Check sheet for the modelled part. Datum: model origin and axes. Units: mm. Face numbers are marked on the shaded views. A direction names the side the tool comes from. Coordinates: 2 decimals unless noted, no trailing zeros. Write each loop counter-clockwise with the first axis right and the second up, starting at its lowest first coordinate (ties: lowest second). Pieces come first, ordered by that corner, then holes. Notation, with made-up numbers: (51, 85.25) - (81, 85.25) arc R33 ccw to (81, 124.25) - close; hole circle Ø8 at (85.25, -13.5). An arc over 180 degrees is marked (long way). Use one line per item in the form item = value. Start each with the question number.
1. Cross-section at A-A on z = 4.5. Record the boundary of the cut face in (x, y).
2. Go/stop test with flat-tipped pins: pin 1 Ø2 at (y, z) = (53.5, 6.5) entering from -X; pin 2 Ø6 at (x, z) = (-11, 10) entering from +Y; pin 3 Ø10 at (x, z) = (-10, 8) entering from -Y. Record where each tip stops, or that it passes through.
3. Cross-section at C-C on y = 6.5. Record the boundary of the cut face in (x, z), then the cut area to 3 significant figures.
4. Tool access check on the marked faces 1, 2 and 3. Record the directions out of +Z, -Z, +X, -X, +Y, -Y that give a thin tool (end or side, any length) a straight path to the whole face; none if there is none.
5. Scan lines: line 1 along X through (y, z) = (51.5, 8); line 2 along Y through (x, z) = (25, 3.75). Record each from-to range of solid material in increasing order.
6. Cross-section at B-B on x = 25. Record the boundary of the cut face in (y, z), then the cut area to 3 significant figures.
```python
from build123d import *

# Parameters (mm, degrees)
F0_W     = 20
F0_H     = 20
F1_DEPTH = 25


with BuildPart() as f1:
    # F0 (on Top) → F1 (new body)
    with BuildSketch(Plane.XY):
        with Locations((10, 10)):
            Rectangle(F0_W, F0_H)
        Polygon((-20, 20), (0, 20), (0, 30), (0, 40), (-20, 40), align=None)
        Polygon((0, 30), (0, 20), (20, 20), (20, 40), (0, 40), align=None)
        with Locations((30, 30)):
            Rectangle(F0_W, F0_H)
        with Locations((10, 50)):
            Rectangle(F0_W, F0_H)
    extrude(amount=F1_DEPTH)


solid = f1.part
```
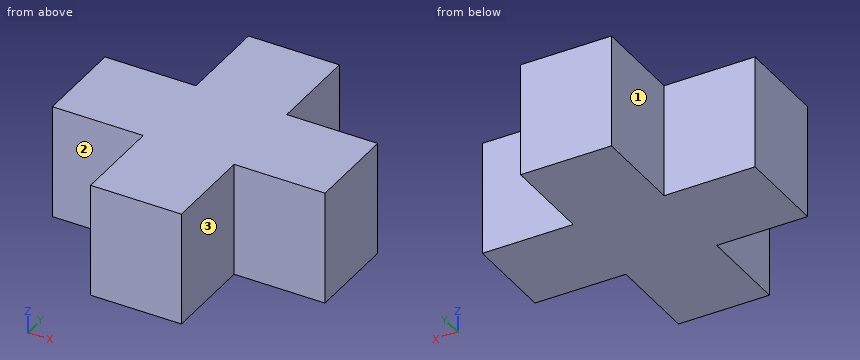
Final values:
q1.outline = (-20, 20) - (0, 20) - (0, 0) - (20, 0) - (20, 20) - (40, 20) - (40, 40) - (20, 40) - (20, 60) - (0, 60) - (0, 40) - (-20, 40) - close
q2.pin_1 = 0
q2.pin_2 = 40
q2.pin_3 = 20
q3.outline = (0, 0) - (20, 0) - (20, 25) - (0, 25) - close
q3.area = 500 mm²
q4.face_1 = +Z, -Z, -X, +Y
q4.face_2 = +Z, -Z, -X, -Y
q4.face_3 = +Z, -Z, +X, -Y
q5.line_1 = 0 to 20
q5.line_2 = 20 to 40
q6.outline = (20, 0) - (40, 0) - (40, 25) - (20, 25) - close
q6.area = 500 mm²
